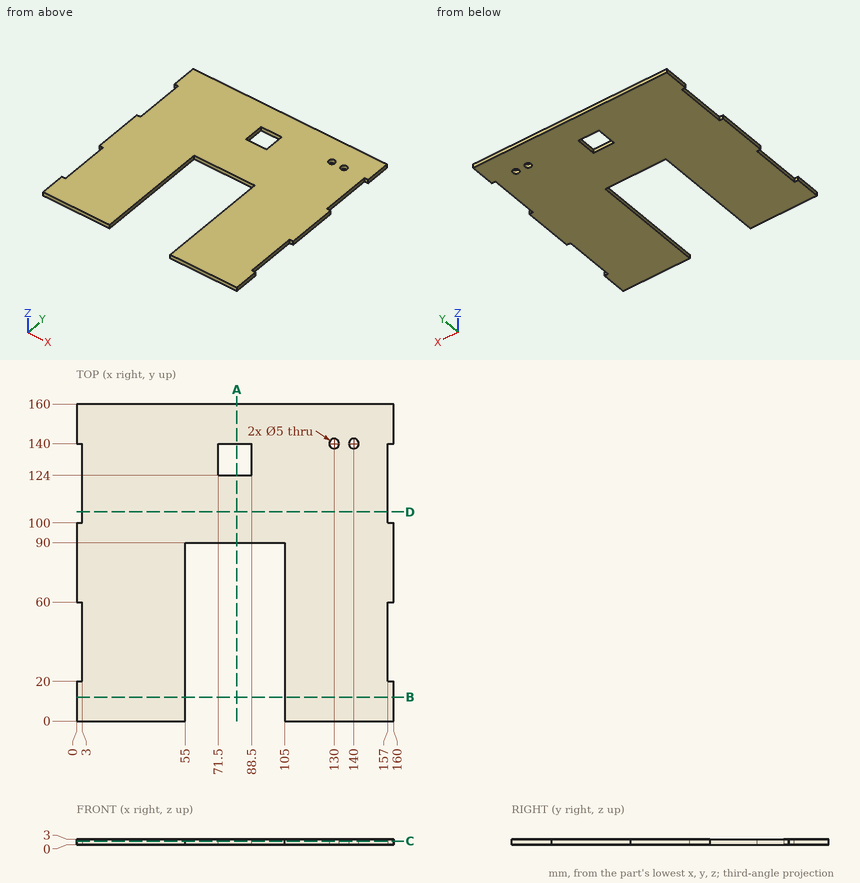
Source: three-view drawing plus pictorial views. Frame: mm from the lowest corner of the part. Coordinates: 2 decimals unless noted, no trailing zeros. Loops run counter-clockwise (first coordinate to the right, second up) from the corner with the lowest first, then second, coordinate; pieces in that order, holes last. Notation, with made-up numbers: (35.25, 60) - (43.25, 60) arc R16 ccw to (43.25, 68) - close; hole circle Ø3 at (-13, 44.5). An arc over 180 degrees is marked (long way). One line per item, written item: value. Start each with the question number.
1. Section B-B (y = 12). Return the cut outline in (x, z), and give its area (3 significant figures).
2. Ray query, L1, parallel to Y at x = 140, z = 1.6; L2, parallel to X at y = 74.5, z = 0.9; L3, parallel to X at y = 49.5, z = 1.05. Return the intervals inside material, ascending.
3. Contact query for flat-ended pins moving along their axis: P1, Ø1.5, axis at y = 41, z = 1, coming from the -X side; P2, Ø1.5, axis at y = 49.5, z = 1.5, coming from the +X side. Output: stop coordinate, or through.
4. Section C-C (z = 1.9). State how many separate pieces and enclosed holes the cut face has, and give its area (3 significant figures).
5. Section D-D (y = 105.5). Return the cut outline in (x, z).
6. Section A-A (x = 81). Return the cut outline in (y, z).
Verdict:
1. outline: (0, 0) - (55, 0) - (55, 3) - (0, 3) - close; (105, 0) - (160, 0) - (160, 3) - (105, 3) - close
1. area: 330 mm2
2. L1: y = 0 to 137.5, 142.5 to 160
2. L2: x = 0 to 55, 105 to 160
2. L3: x = 3 to 55, 105 to 157
3. P1: stops at x = 3
3. P2: stops at x = 157
4. separate pieces: 1
4. enclosed holes: 3
4. area: 20,300 mm2
5. outline: (3, 0) - (157, 0) - (157, 3) - (3, 3) - close
6. outline: (90, 0) - (124, 0) - (124, 3) - (90, 3) - close; (140, 0) - (160, 0) - (160, 3) - (140, 3) - close
